```python
from build123d import *

# Parameters (mm, degrees)
SKETCH1_R           = 17
SKETCH1_R_2         = 10.32
BOSS_EXTRUDE1_DEPTH = 2
SKETCH5_R           = 15.24
SKETCH5_R_2         = 13.99
CUT_EXTRUDE1_DEPTH  = 0.4
SKETCH6_R           = 12.23
SKETCH6_R_2         = 12.08
CUT_EXTRUDE2_DEPTH  = 0.4


with BuildPart() as part:
    # Sketch1 → Boss-Extrude1 (new body)
    with BuildSketch(Plane(origin=(0, 0, 0), x_dir=(0, 0, -1), z_dir=(1, 0, 0))):
        Circle(SKETCH1_R)
        Circle(SKETCH1_R_2, mode=Mode.SUBTRACT)
    extrude(amount=BOSS_EXTRUDE1_DEPTH)

    # Sketch4 → Revolve3 (revolve)
    with BuildSketch(Plane(origin=(0, 0, 0), x_dir=(1, 0, 0), z_dir=(0, 1, 0))):
        with BuildLine():
            Line((9.2, 13.99), (9.2, 12.23))
            Line((9.2, 12.23), (8, 12.23))
            ThreePointArc((8, 12.23), (5.6, 12.89), (3.2, 12.23))
            Line((3.2, 12.23), (2, 12.23))
            Line((2, 12.23), (2, 13.99))
            Line((2, 13.99), (3.199999942, 13.99))
            ThreePointArc((3.199999942, 13.99), (5.599998351, 14.65), (7.999996761, 13.99))
            Line((7.999996761, 13.99), (9.2, 13.99))
        make_face()
    revolve(axis=Axis((2, 0, 0), (-1, 0, 0)))

    # Sketch5 → Cut-Extrude1 (cut)
    with BuildSketch(Plane(origin=(2, 0, 0), x_dir=(0, 0, -1), z_dir=(1, 0, 0))):
        Circle(SKETCH5_R)
        Circle(SKETCH5_R_2, mode=Mode.SUBTRACT)
    extrude(amount=-CUT_EXTRUDE1_DEPTH, mode=Mode.SUBTRACT)

    # Sketch6 → Cut-Extrude2 (cut)
    with BuildSketch(Plane(origin=(2, 0, 0), x_dir=(0, 0, -1), z_dir=(1, 0, 0))):
        Circle(SKETCH6_R)
        Circle(SKETCH6_R_2, mode=Mode.SUBTRACT)
    extrude(amount=-CUT_EXTRUDE2_DEPTH, mode=Mode.SUBTRACT)


solid = part.part
```
Geometry check sheet. Reference: the model listing, model coordinates, mm. A direction names the side the tool comes from. Coordinates: 2 decimals unless noted, no trailing zeros. Order: outer loops, then holes, each group sorted by start corner. A loop starts at its lowest first (then second) coordinate and runs counter-clockwise, first axis right, second up. Notation, with made-up numbers: M -7,85.25 L 7,85.25 A21 cw 7,117.25 Z; hole C -10.5,-30 d5. An arc over 180 degrees is marked long. One line per question, with ' | ' between items. Start each with the question number.
Item 1: Draft check along X on faces 1 (the flat face through (0, -11, 0)), 2 (the cylindrical face through (0.986, 14.334, -9.139)), 3 (the flat face through (9.2, 12.4, 0.1)), 4 (the flat face through (1.6, -4.4, -13.5)). Enter one of: pulls with the +X half, pulls with the -X half, needs draft (parallel to the pull), parting line crosses it, or undercut.
Item 2: Set-up check for faces 5 (the cylindrical face through (0.99, -6.28, 8.19)), 6 (the cylindrical face through (1.8, -14.88, 3.3)): record each of +Z, -Z, +X, -X, +Y, -Y from which the full face is reachable in a straight line by a thin tool's end or side.
Item 3: Material ranges on L1, parallel to Y at x = 8.4, z = 0; L2, parallel to X at y = -8.5, z = -6.5; L3, parallel to X at y = -11, z = 6, recorded low to high. Write a range as [from, to].
Item 4: Cross-section at C-C on x = 2.75. Enter the section's corners in (y, z).
Item 5: Gauge pin test, flat ends, axial feed: pin 1 (12 mm diameter, centred on y = 3, z = -4.5, fed in from +X); pin 2 (3 mm diameter, centred on x = 2.5, z = -3, fed in from +Y); pin 3 (14.5 mm diameter, centred on y = 0, z = 0, fed in from +X); pin 4 (1.5 mm diameter, centred on x = 4, y = 10.5, fed in from +Z). Record the tip position at first contact, or that the pin passes through.
Findings:
1) face 1: pulls with the -X half | face 2: needs draft | face 3: pulls with the +X half | face 4: undercut
2) face 5: +X, -X | face 6: +X
3) L1: y = [-13.99, -12.23], [12.23, 13.99] | L2: x = [0, 2] | L3: x = [0, 3.8], [7.4, 9.2]
4) outline: C 0,0 d27.98; hole C 0,0 d24.46
5) pin 1: stops at x = 2 | pin 2: stops at y = 16.93 | pin 3: passes through | pin 4: stops at z = 10.63
